```python
from build123d import *

# Parameters (mm, degrees)
SKETCH_1_W           = 174.15
SKETCH_1_H           = 108
EXTRUDE_1_DEPTH      = 63
CUT_EXTRUDE_2_DEPTH  = 174.15
CUT_EXTRUDE_3_REACH  = 122.279
SKETCH_6_W           = 2
SKETCH_6_H           = 108
SKETCH_7_W           = 96
SKETCH_7_H           = 50.25
CUT_EXTRUDE_5_DEPTH  = 168.15
SKETCH_8_W           = 87.5
SKETCH_8_H           = 4.75
CUT_EXTRUDE_6_DEPTH  = 168.15
SKETCH_10_W          = 168.15
SKETCH_10_H          = 87.5
CUT_EXTRUDE_8_DEPTH  = 59
SKETCH_12_W          = 168.15
SKETCH_12_H          = 96
EXTRUDE_2_DEPTH      = 2
SKETCH_15_W          = 25
SKETCH_15_H          = 70
SKETCH_15_W_2        = 55
SKETCH_15_H_2        = 20
SKETCH_15_W_3        = 44.398131355
SKETCH_15_H_3        = 87.5
CUT_EXTRUDE_9_DEPTH  = 2
SKETCH_16_W          = 25
SKETCH_16_H          = 96
SKETCH_16_W_2        = 32.283516817
CUT_EXTRUDE_10_DEPTH = 2
SKETCH_17_W          = 2
SKETCH_17_H          = 96
EXTRUDE_3_DEPTH      = 5
SKETCH_18_W          = 2
SKETCH_18_H          = 87.5
EXTRUDE_4_DEPTH      = 5
SKETCH_19_W          = 100
SKETCH_19_H          = 18
CUT_EXTRUDE_11_DEPTH = 6
CUT_EXTRUDE_12_REACH = 154.365
EXTRUDE_5_REACH      = 154.365
SKETCH_23_W          = 65.205598619
SKETCH_23_H          = 48.744694075
CUT_EXTRUDE_13_DEPTH = 2
CUT_EXTRUDE_START    = -63
CUT_EXTRUDE_14_DEPTH = 63
SKETCH_28_W          = 2
SKETCH_28_H          = 4.25
EXTRUDE_6_DEPTH      = 4.75
SKETCH_31_W          = 13
SKETCH_31_H          = 55
CUT_EXTRUDE_15_DEPTH = 10
SKETCH_34_W          = 103.070926165
SKETCH_34_H          = 3
CUT_EXTRUDE_16_DEPTH = 143.15


with BuildPart() as part:
    # 스케치1 → 보스-돌출1 (new body)
    with BuildSketch(Plane(origin=(0, 0, 0), x_dir=(1, 0, 0), z_dir=(0, 1, 0))):
        Rectangle(SKETCH_1_W, SKETCH_1_H)
    extrude(amount=EXTRUDE_1_DEPTH)

    # 스케치5 → 컷-돌출2 (cut)
    with BuildSketch(Plane.ZY.offset(87.075)):
        Polygon((-48, 0), (-47.75, 0), (-47.75, 2.75), (-45.75, 2.75), (-45.75, 4.75), (-52.25, 4.75), (-52.25, 2.75), (-50.25, 2.75), (-50.25, 0), (-50, 0), (-50, 3), (-52, 3), (-52, 4.5), (-46, 4.5), (-46, 3), (-48, 3), align=None)
        Polygon((-50, 0), (-48, 0), (-48, 3), (-46, 3), (-46, 4.5), (-52, 4.5), (-52, 3), (-50, 3), align=None)
        Polygon((50, 3), (50, 0), (50.25, 0), (50.25, 2.75), (52.25, 2.75), (52.25, 4.75), (45.75, 4.75), (45.75, 2.75), (47.75, 2.75), (47.75, 0), (48, 0), (48, 3), (46, 3), (46, 4.5), (52, 4.5), (52, 3), align=None)
        Polygon((48, 0), (50, 0), (50, 3), (52, 3), (52, 4.5), (46, 4.5), (46, 3), (48, 3), align=None)
    extrude(amount=-CUT_EXTRUDE_2_DEPTH, mode=Mode.SUBTRACT)

    # 컷-돌출3: up to this face of the body (flat: up to its plane)
    cut_extrude_3_end = Plane(part.part.faces().sort_by_distance((0, 4.75, 49))[0])
    # 스케치6 → 컷-돌출3 (cut, up to the picked face)
    with BuildSketch(Plane.XZ, mode=Mode.PRIVATE) as cut_extrude_3_sk1:
        with Locations((-86.075, 0)):
            Rectangle(SKETCH_6_W, SKETCH_6_H)
    cut_extrude_3_tool1 = split(extrude(cut_extrude_3_sk1.sketch, amount=-CUT_EXTRUDE_3_REACH, mode=Mode.PRIVATE), bisect_by=cut_extrude_3_end, keep=Keep.BOTH, mode=Mode.PRIVATE)
    add(cut_extrude_3_tool1.solids().sort_by(Axis((-86.075, 0, 0), (0, 1, 0)))[0], mode=Mode.SUBTRACT)

    # 스케치7 → 컷-돌출5 (cut)
    with BuildSketch(Plane(origin=(87.075, 0, 0), x_dir=(0, 0, -1), z_dir=(1, 0, 0))):
        with Locations((0, 31.875)):
            Rectangle(SKETCH_7_W, SKETCH_7_H)
    extrude(amount=-CUT_EXTRUDE_5_DEPTH, mode=Mode.SUBTRACT)

    # 스케치8 → 컷-돌출6 (cut)
    with BuildSketch(Plane(origin=(87.075, 0, 0), x_dir=(0, 0, -1), z_dir=(1, 0, 0))):
        with Locations((0, 4.375)):
            Rectangle(SKETCH_8_W, SKETCH_8_H)
    extrude(amount=-CUT_EXTRUDE_6_DEPTH, mode=Mode.SUBTRACT)

    # 스케치10 → 컷-돌출8 (cut)
    with BuildSketch(Plane(origin=(0, 2, 0), x_dir=(1, 0, 0), z_dir=(0, 1, 0))):
        with Locations((3, 0)):
            Rectangle(SKETCH_10_W, SKETCH_10_H)
    extrude(amount=CUT_EXTRUDE_8_DEPTH, mode=Mode.SUBTRACT)

    # 스케치12 → 보스-돌출2 (add)
    with BuildSketch(Plane(origin=(0, 24, 0), x_dir=(-1, 0, 0), z_dir=(0, -1, 0))):
        with Locations((-3, 0)):
            Rectangle(SKETCH_12_W, SKETCH_12_H)
    extrude(amount=EXTRUDE_2_DEPTH)

    # 스케치15 → 컷-돌출9 (cut)
    with BuildSketch(Plane(origin=(0, 2, 0), x_dir=(1, 0, 0), z_dir=(0, 1, 0))):
        with Locations((-68.575, 8.75)):
            Rectangle(SKETCH_15_W, SKETCH_15_H)
        with Locations((-9.233175572, -33.75)):
            Rectangle(SKETCH_15_W_2, SKETCH_15_H_2)
        with Locations((64.875934323, 0)):
            Rectangle(SKETCH_15_W_3, SKETCH_15_H_3)
    extrude(amount=-CUT_EXTRUDE_9_DEPTH, mode=Mode.SUBTRACT)

    # 스케치16 → 컷-돌출10 (cut)
    with BuildSketch(Plane(origin=(0, 24, 0), x_dir=(1, 0, 0), z_dir=(0, 1, 0))):
        with Locations((-68.575, 0)):
            Rectangle(SKETCH_16_W, SKETCH_16_H)
        with Locations((70.933241592, 0)):
            Rectangle(SKETCH_16_W_2, SKETCH_16_H)
    extrude(amount=-CUT_EXTRUDE_10_DEPTH, mode=Mode.SUBTRACT)

    # 스케치17 → 보스-돌출3 (add)
    with BuildSketch(Plane(origin=(0, 24, 0), x_dir=(1, 0, 0), z_dir=(0, 1, 0))):
        with Locations((-55.075, 0)):
            Rectangle(SKETCH_17_W, SKETCH_17_H)
    extrude(amount=EXTRUDE_3_DEPTH)

    # 스케치18 → 보스-돌출4 (add)
    with BuildSketch(Plane(origin=(0, 2, 0), x_dir=(1, 0, 0), z_dir=(0, 1, 0))):
        with Locations((-55.075, 0)):
            Rectangle(SKETCH_18_W, SKETCH_18_H)
    extrude(amount=EXTRUDE_4_DEPTH)

    # 스케치19 → 컷-돌출11 (cut)
    with BuildSketch(Plane(origin=(0, 0, 48), x_dir=(-1, 0, 0), z_dir=(0, 0, -1))):
        with Locations((4.075, 38)):
            Rectangle(SKETCH_19_W, SKETCH_19_H)
    extrude(amount=-CUT_EXTRUDE_11_DEPTH, mode=Mode.SUBTRACT)

    # 컷-돌출12: up to this face of the body (flat: up to its plane)
    cut_extrude_12_end = Plane(part.part.faces().sort_by_distance((0.074595533, 31.525240719, -54))[0])
    # 스케치20 → 컷-돌출12 (cut, up to the picked face)
    with BuildSketch(Plane.XY.offset(54), mode=Mode.PRIVATE) as cut_extrude_12_sk1:
        Polygon((-87.075, 4.75), (-54.075, 63), (-87.075, 63), align=None)
    cut_extrude_12_tool1 = split(extrude(cut_extrude_12_sk1.sketch, amount=-CUT_EXTRUDE_12_REACH, mode=Mode.PRIVATE), bisect_by=cut_extrude_12_end, keep=Keep.BOTH, mode=Mode.PRIVATE)
    add(cut_extrude_12_tool1.solids().sort_by(Axis((-76.075, 43.583333, 54), (0, 0, -1)))[0], mode=Mode.SUBTRACT)

    # 보스-돌출5: up to this face of the body (flat: up to its plane)
    extrude_5_end = Plane(part.part.faces().sort_by_distance((7.392919772, 30.366402897, -54))[0])
    # 스케치21 → 보스-돌출5 (add, up to the picked face)
    with BuildSketch(Plane.XY.offset(54), mode=Mode.PRIVATE) as extrude_5_sk1:
        Polygon((-87.075, 4.75), (-84.776349095, 4.75), (-51.776349095, 63), (-54.075, 63), align=None)
    extrude_5_tool1 = split(extrude(extrude_5_sk1.sketch, amount=-EXTRUDE_5_REACH, mode=Mode.PRIVATE), bisect_by=extrude_5_end, keep=Keep.BOTH, mode=Mode.PRIVATE)
    add(extrude_5_tool1.solids().sort_by(Axis((-69.425675, 33.875, 54), (0, 0, -1)))[0])

    # 스케치23 → 컷-돌출13 (cut)
    with BuildSketch(Plane(origin=(0, 63, 0), x_dir=(1, 0, 0), z_dir=(0, 1, 0))):
        with Locations((-5.140341164, 12.481591832)):
            Rectangle(SKETCH_23_W, SKETCH_23_H)
    extrude(amount=-CUT_EXTRUDE_13_DEPTH, mode=Mode.SUBTRACT)

    # 스케치26 → 컷-돌출14 (cut)
    with BuildSketch(Plane(origin=(0, 63, 0), x_dir=(1, 0, 0), z_dir=(0, 1, 0)).offset(CUT_EXTRUDE_START)):
        Polygon((82.075, 52), (85.075, 52), (85.075, 48), (87.075, 48), (87.075, -48), (85.075, -48), (85.075, -52), (82.075, -52), align=None)
    extrude(amount=CUT_EXTRUDE_14_DEPTH, mode=Mode.SUBTRACT)

    # 스케치28 → 보스-돌출6 (add)
    with BuildSketch(Plane.XZ.offset(-4.75)):
        with Locations((86.075, 50.125)):
            Rectangle(SKETCH_28_W, SKETCH_28_H)
        with Locations((86.075, -50.125)):
            Rectangle(SKETCH_28_W, SKETCH_28_H)
    extrude(amount=EXTRUDE_6_DEPTH)

    # 스케치31 → 컷-돌출15 (cut)
    with BuildSketch(Plane(origin=(0, 63, 0), x_dir=(1, 0, 0), z_dir=(0, 1, 0))):
        with Locations((75.575, 0)):
            Rectangle(SKETCH_31_W, SKETCH_31_H)
    extrude(amount=-CUT_EXTRUDE_15_DEPTH, mode=Mode.SUBTRACT)

    # 스케치34 → 컷-돌출16 (cut)
    with BuildSketch(Plane(origin=(87.075, 0, 0), x_dir=(0, 0, -1), z_dir=(1, 0, 0))):
        with Locations((-0.464536917, 23.5)):
            Rectangle(SKETCH_34_W, SKETCH_34_H)
    extrude(amount=-CUT_EXTRUDE_16_DEPTH, mode=Mode.SUBTRACT)


solid = part.part
```
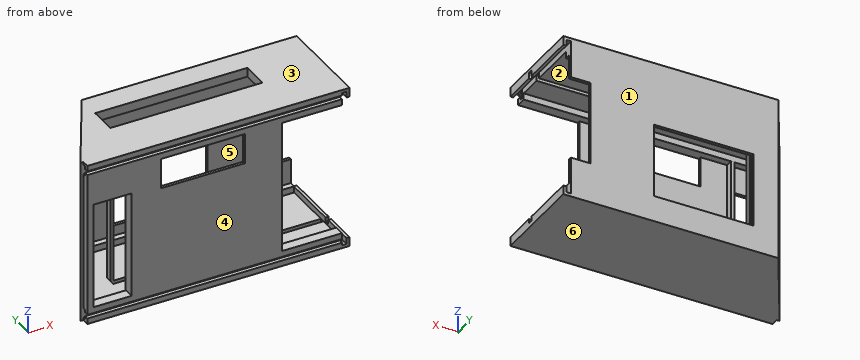
Verification items for the finished model (mm, model axes). Face numbers are marked on the shaded views. A direction names the side the tool comes from. Coordinates: 2 decimals unless noted, no trailing zeros. Order: outer loops, then holes, each group sorted by start corner. A loop starts at its lowest first (then second) coordinate and runs counter-clockwise, first axis right, second up. Notation, with made-up numbers: (20.5, 67.25) - (24.5, 67.25) arc R15 cw to (24.5, 87.25) - close; hole circle Ø1 at (29, 22.25). An arc over 180 degrees is marked (long way). Return JSON: item names as keys, results as strings.
(1) Go/stop test with flat-tipped pins: pin 1 (1.5 mm diameter, centred on x = -27.5, y = 39.5, fed in from +Z); pin 2 (6 mm diameter, centred on x = 16.5, z = -30.5, fed in from +Y); pin 3 (6 mm diameter, centred on x = -63, z = -8, fed in from +Y). Record where each tip stops, or that it passes through.
Filled sheet:
{"pin 1": "stops at z = -48", "pin 2": "stops at y = 2", "pin 3": "stops at y = 52.54"}
(2) Access from +Z, -Z, +X, -X, +Y, -Y to the whole of each face (thin tool, end or side, straight path). Record for the marked faces 5 and 6.
Filled sheet:
{"face 5": "+X", "face 6": "-Z, +X, -X, +Y, -Y"}
(3) Mould release check, pull along Y, two halves, no side actions. Record for the marked faces 1, 2, 3 and 4: pulls with the +Y half, pulls with the -Y half, needs draft (parallel to the pull), parting line crosses it, or undercut.
Filled sheet:
{"face 1": "pulls with the +Y half", "face 2": "undercut", "face 3": "needs draft", "face 4": "pulls with the -Y half"}
(4) Thickness scan on line 1 along Z through (x, y) = (7, 49.5); line 2 along Y through (x, z) = (-10.5, -37); line 3 along X through (y, z) = (4.5, 31) (3 decimals). Record the ranges inside material, lowest first.
Filled sheet:
{"line 1": "z = -54 to -48, 48 to 54", "line 2": "y = 0 to 2, 61 to 63", "line 3": "x = -85.075 to -81.075, -56.075 to -54.075"}
(5) Section check C-C, the plane y = 40. Record the cut outline in (x, z) (3 decimals), and give its area (3 significant figures).
Filled sheet:
{"outline": "(-67.105, -54) - (87.075, -54) - (87.075, -48) - (85.075, -48) - (85.075, -52) - (82.075, -52) - (82.075, -48) - (-64.806, -48) - (-64.806, 48) - (-54.075, 48) - (-54.075, 54) - (-67.105, 54) - close; (45.925, 48) - (82.075, 48) - (82.075, 52) - (85.075, 52) - (85.075, 48) - (87.075, 48) - (87.075, 54) - (45.925, 54) - close", "area": "1,450 mm^2"}
(6) Section check B-B, the plane z = 41. Record the cut outline in (x, y) (3 decimals).
Filled sheet:
{"outline": "(-87.075, 4.75) - (-85.075, 4.75) - (-85.075, 0) - (-36.733, 0) - (-36.733, 2) - (-54.075, 2) - (-54.075, 7) - (-56.075, 7) - (-56.075, 2) - (-81.075, 2) - (-81.075, 11.283) - (-52.909, 61) - (82.075, 61) - (82.075, 63) - (-54.075, 63) - close; (-56.075, 25) - (-54.075, 25) - (-54.075, 29) - (-56.075, 29) - close; (18.267, 0) - (42.677, 0) - (42.677, 2) - (18.267, 2) - close"}
(7) Section check A-A, the plane z = -12. Record the cut outline in (x, y) (3 decimals).
Filled sheet:
{"outline": "(-87.075, 4.75) - (-85.075, 4.75) - (-85.075, 0) - (-81.075, 0) - (-81.075, 11.283) - (-52.909, 61) - (-37.743, 61) - (-37.743, 63) - (-54.075, 63) - close; (-56.075, 0) - (42.677, 0) - (42.677, 2) - (-54.075, 2) - (-54.075, 7) - (-56.075, 7) - close; (-56.075, 25) - (-54.075, 25) - (-54.075, 29) - (-56.075, 29) - close; (27.462, 61) - (69.075, 61) - (69.075, 63) - (27.462, 63) - close"}
(8) Section check D-D, the plane x = -27. Give the number of separate pieces and of enclosed holes in the cut face, and give its area (3 significant figures).
Filled sheet:
{"separate pieces": "3", "enclosed holes": "0", "area": "908 mm^2"}
